```python
from build123d import *

# Parameters (mm, degrees)
PAD_DEPTH       = 49.5
CHAMFER_SIZE    = 1.5
CHAMFER001_SIZE = 0.5
CHAMFER002_SIZE = 1
SKETCH001_R     = 2.5
POCKET_DEPTH    = 5


with BuildPart() as part:
    # Sketch → Pad (new body)
    with BuildSketch(Plane.XY):
        Polygon((0, 0), (14.25, 0), (14.25, 6), (11.75, 6), (11.75, 9), (14.25, 9), (14.25, 12.5), (17.25, 12.5), (17.25, -3), (0, -3), align=None)
    pad = extrude(amount=PAD_DEPTH)

    # Mirrored: Pad across Sketch V_Axis
    add(pad.mirror(Plane(origin=(0, 0, 0), x_dir=(0, 0, 1), z_dir=(1, 0, 0))))

    # Chamfer
    chamfer_edges = [part.edges().sort_by_distance(p)[0] for p in [
        (-17.25, 12.5, 24.75),
        (17.25, 12.5, 24.75),
    ]]
    chamfer(chamfer_edges, length=CHAMFER_SIZE)

    # Chamfer001
    chamfer001_edges = [part.edges().sort_by_distance(p)[0] for p in [
        (-11.75, 9, 24.75),
        (-11.75, 6, 24.75),
        (11.75, 9, 24.75),
        (11.75, 6, 24.75),
    ]]
    chamfer(chamfer001_edges, length=CHAMFER001_SIZE)

    # Chamfer002
    chamfer002_edges = [part.edges().sort_by_distance(p)[0] for p in [
        (-17.25, -3, 24.75),
        (17.25, -3, 24.75),
    ]]
    chamfer(chamfer002_edges, length=CHAMFER002_SIZE)

    # Sketch001 (on Face9 of Chamfer002) → Pocket (cut)
    with BuildSketch(Plane(origin=(0, 0, 0), x_dir=(-1, 0, 0), z_dir=(0, 1, 0))):
        with Locations((-9, 3.5)):
            Circle(SKETCH001_R)
        with Locations((-9, 9.5)):
            Circle(SKETCH001_R)
        with Locations((-9, 15.5)):
            Circle(SKETCH001_R)
        with Locations((-9, 21.5)):
            Circle(SKETCH001_R)
        with Locations((-9, 27.5)):
            Circle(SKETCH001_R)
        with Locations((-9, 33.5)):
            Circle(SKETCH001_R)
        with Locations((-9, 39.5)):
            Circle(SKETCH001_R)
        with Locations((-9, 45.5)):
            Circle(SKETCH001_R)
        with Locations((-3, 3.5)):
            Circle(SKETCH001_R)
        with Locations((-3, 9.5)):
            Circle(SKETCH001_R)
        with Locations((-3, 15.5)):
            Circle(SKETCH001_R)
        with Locations((-3, 21.5)):
            Circle(SKETCH001_R)
        with Locations((-3, 27.5)):
            Circle(SKETCH001_R)
        with Locations((-3, 33.5)):
            Circle(SKETCH001_R)
        with Locations((-3, 39.5)):
            Circle(SKETCH001_R)
        with Locations((-3, 45.5)):
            Circle(SKETCH001_R)
        with Locations((3, 3.5)):
            Circle(SKETCH001_R)
        with Locations((3, 9.5)):
            Circle(SKETCH001_R)
        with Locations((3, 15.5)):
            Circle(SKETCH001_R)
        with Locations((3, 21.5)):
            Circle(SKETCH001_R)
        with Locations((3, 27.5)):
            Circle(SKETCH001_R)
        with Locations((3, 33.5)):
            Circle(SKETCH001_R)
        with Locations((3, 39.5)):
            Circle(SKETCH001_R)
        with Locations((3, 45.5)):
            Circle(SKETCH001_R)
        with Locations((9, 3.5)):
            Circle(SKETCH001_R)
        with Locations((9, 9.5)):
            Circle(SKETCH001_R)
        with Locations((9, 15.5)):
            Circle(SKETCH001_R)
        with Locations((9, 21.5)):
            Circle(SKETCH001_R)
        with Locations((9, 27.5)):
            Circle(SKETCH001_R)
        with Locations((9, 33.5)):
            Circle(SKETCH001_R)
        with Locations((9, 39.5)):
            Circle(SKETCH001_R)
        with Locations((9, 45.5)):
            Circle(SKETCH001_R)
    extrude(amount=-POCKET_DEPTH, mode=Mode.SUBTRACT)


solid = part.part
```
For this review, take the finished solid that the model builds, in its own axes (mm). A direction names the side the tool comes from. Round coordinates to 2 decimals unless told otherwise and drop trailing zeros. Order: outer loops, then holes, each group sorted by start corner. A loop starts at its lowest first (then second) coordinate and runs counter-clockwise, first axis right, second up.
Q1. We need section A-A, the plane y = 0.5. Give the boundary of the cut face in (x, z).
Findings below:
outline: (-17.25, 0) - (-14.25, 0) - (-14.25, 49.5) - (-17.25, 49.5) - close; (14.25, 0) - (17.25, 0) - (17.25, 49.5) - (14.25, 49.5) - close
Q2. Insertion check: P1, Ø8, axis at x = -3, z = 33.5, coming from the +Y side. The pin has a flat end and moves straight along its axis. Give the tip position at first contact, or say it passes through.
Findings below:
P1: stops at y = 0
Q3. Machinability: for faces 1 (the flat face through (16.76, -2.49, 24.4)), 2 (the flat face through (-14.25, 3, 24)), 3 (the flat face through (-14.25, 11, 24)), which of the approach directions +Z, -Z, +X, -X, +Y, -Y give a long, thin tool a straight path to every point of the face, cutting with its end or side? Answer none if there is none.
Findings below:
face 1: +Z, -Z, +X, -Y
face 2: +Z, -Z
face 3: +Z, -Z, +Y
Q4. Wall thickness on line 1 (Y direction, x = -13, z = 46); line 2 (X direction, y = 1, z = 20.5); line 3 (Y direction, x = -3.5, z = 6.5): over which ranges is each line inside the solid? List them lowest first.
Findings below:
line 1: y = -3 to 0, 6 to 9
line 2: x = -17.25 to -14.25, 14.25 to 17.25
line 3: y = -3 to 0
Q5. Mouldability with a two-part tool opening along Z and no side actions: class faces 4 (the cylindrical face through (3.54, -1.48, 37.06)), 5 (the cylindrical face through (-3, -1, 6)), 6 (the flat face through (-0.2, -0.3, 49.5)), 7 (the flat face through (13, 9, 24)) as pulls with the +Z half, pulls with the -Z half, needs draft (parallel to the pull), parting line crosses it, or undercut.
Findings below:
face 4: undercut
face 5: undercut
face 6: pulls with the +Z half
face 7: needs draft
Q6. We need section B-B, the plane x = -3. State how many separate pieces and enclosed holes the cut face has, plus the area to 3 significant figures.
Findings below:
separate pieces: 9
enclosed holes: 0
area: 28.5 mm2
